Read the model definition and answer for the solid it produces. Units are mm, in the model's axes. Face numbers are marked on the shaded views. A direction names the side the tool comes from. Give positions to 0.01 mm unless a question says otherwise; leave off trailing zeros. Order: outer loops, then holes, each group sorted by start corner. A loop starts at its lowest first (then second) coordinate and runs counter-clockwise, first axis right, second up. Notation, with made-up numbers: (53, 28.25) -> (68, 28.25) arc R29 ccw to (68, 56.25) -> close; hole circle Ø1 at (72.25, 20). An arc over 180 degrees is marked (long way). One line per question, with ' | ' between items. Start each with the question number.
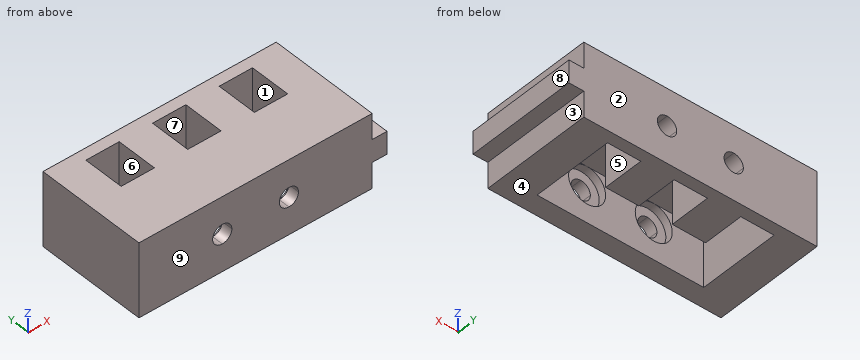
```python
from build123d import *

# Parameters (mm, degrees)
SKETCH_1_W          = 63
SKETCH_1_H          = 30
SKETCH_1_W_2        = 9
SKETCH_1_H_2        = 11
EXTRUDE_2_DEPTH     = 20
SKETCH_2_W          = 9
SKETCH_2_H          = 11
CUT_EXTRUDE_1_DEPTH = 15
SKETCH_3_W          = 9
SKETCH_3_H          = 11
EXTRUDE_3_DEPTH     = 15
CUT_EXTRUDE_2_DEPTH = 100
SKETCH_6_R          = 5
CUT_EXTRUDE_3_DEPTH = 2
SKETCH_7_W          = 3.05
SKETCH_7_H          = 15
EXTRUDE_4_DEPTH     = 4


with BuildPart() as part:
    # 草图1 → 凸台-拉伸2 (new body)
    with BuildSketch(Plane.XY):
        with Locations((18.5, 15)):
            Rectangle(SKETCH_1_W, SKETCH_1_H)
        with Locations((18.5, 21.5)):
            Rectangle(SKETCH_1_W_2, SKETCH_1_H_2, mode=Mode.SUBTRACT)
        with Locations((36.5, 21.5)):
            Rectangle(SKETCH_1_W_2, SKETCH_1_H_2, mode=Mode.SUBTRACT)
        with Locations((0.5, 21.5)):
            Rectangle(SKETCH_1_W_2, SKETCH_1_H_2, mode=Mode.SUBTRACT)
    extrude(amount=EXTRUDE_2_DEPTH)

    # 草图2 → 切除-拉伸1 (cut)
    with BuildSketch(Plane(origin=(0, 0, 0), x_dir=(-1, 0, 0), z_dir=(0, 0, -1))):
        Polygon((-50, 16), (-50, 5), (4, 5), (4, 16), (-5, 16), (-14, 16), (-23, 16), (-32, 16), (-41, 16), align=None)
        with Locations((8.5, 10.5)):
            Rectangle(SKETCH_2_W, SKETCH_2_H)
    extrude(amount=-CUT_EXTRUDE_1_DEPTH, mode=Mode.SUBTRACT)

    # 草图3 → 凸台-拉伸3 (add)
    with BuildSketch(Plane(origin=(0, 0, 0), x_dir=(-1, 0, 0), z_dir=(0, 0, -1))):
        with Locations((-45.5, 10.5)):
            Rectangle(SKETCH_3_W, SKETCH_3_H)
        with Locations((8.5, 10.5)):
            Rectangle(SKETCH_3_W, SKETCH_3_H)
    extrude(amount=-EXTRUDE_3_DEPTH)

    # 草图5 → 切除-拉伸2 (cut)
    with BuildSketch(Plane.XZ):
        with BuildLine():
            ThreePointArc((27.5, 12.6), (25.661522369, 11.838477631), (24.9, 10))
            Line((24.9, 10), (27.5, 10))
            Line((27.5, 10), (27.5, 12.6))
        make_face()
        with BuildLine():
            Line((27.5, 10), (24.9, 10))
            ThreePointArc((24.9, 10), (25.661522369, 8.161522369), (27.5, 7.4))
            Line((27.5, 7.4), (27.5, 10))
        make_face()
        with BuildLine():
            Line((30.1, 10), (27.5, 10))
            Line((27.5, 10), (27.5, 7.4))
            ThreePointArc((27.5, 7.4), (29.338477631, 8.161522369), (30.1, 10))
        make_face()
        with BuildLine():
            Line((27.5, 12.6), (27.5, 10))
            Line((27.5, 10), (30.1, 10))
            ThreePointArc((30.1, 10), (29.338477631, 11.838477631), (27.5, 12.6))
        make_face()
        with BuildLine():
            Line((9.5, 10), (9.5, 7.4))
            ThreePointArc((9.5, 7.4), (11.338477631, 8.161522369), (12.1, 10))
            Line((12.1, 10), (9.5, 10))
        make_face()
        with BuildLine():
            Line((9.5, 12.6), (9.5, 10))
            Line((9.5, 10), (12.1, 10))
            ThreePointArc((12.1, 10), (11.338477631, 11.838477631), (9.5, 12.6))
        make_face()
        with BuildLine():
            ThreePointArc((6.9, 10), (7.661522369, 8.161522369), (9.5, 7.4))
            Line((9.5, 7.4), (9.5, 10))
            Line((9.5, 10), (6.9, 10))
        make_face()
        with BuildLine():
            Line((6.9, 10), (9.5, 10))
            Line((9.5, 10), (9.5, 12.6))
            ThreePointArc((9.5, 12.6), (7.661522369, 11.838477631), (6.9, 10))
        make_face()
    extrude(amount=-CUT_EXTRUDE_2_DEPTH, mode=Mode.SUBTRACT)

    # 草图6 → 切除-拉伸3 (cut)
    with BuildSketch(Plane(origin=(0, 5, 0), x_dir=(1, 0, 0), z_dir=(0, 1, 0))):
        with Locations(Location((9.5, -10, 0), (0, 0, 270))):
            Circle(SKETCH_6_R)
        with Locations(Location((27.5, -10, 0), (0, 0, 270))):
            Circle(SKETCH_6_R)
    extrude(amount=-CUT_EXTRUDE_3_DEPTH, mode=Mode.SUBTRACT)

    # 草图7 → 凸台-拉伸4 (add)
    with BuildSketch(Plane(origin=(50, 0, 0), x_dir=(0, 0, -1), z_dir=(1, 0, 0))):
        with Locations((-8.475, 22.5)):
            Rectangle(SKETCH_7_W, SKETCH_7_H)
        with Locations((-11.525, 22.5)):
            Rectangle(SKETCH_7_W, SKETCH_7_H)
        with Locations((-11.525, 7.5)):
            Rectangle(SKETCH_7_W, SKETCH_7_H)
        with Locations((-8.475, 7.5)):
            Rectangle(SKETCH_7_W, SKETCH_7_H)
    extrude(amount=EXTRUDE_4_DEPTH)


solid = part.part
```
Q1. A cutting plane is placed at C-C, the plane z = 1. Determine the outline of the cut face in (x, y).
Q2. Given P1, Ø2, axis at y = 7, z = 2, coming from the +X side; P2, Ø3, axis at x = 52.5, y = 13.5, coming from the -Z side; P3, Ø1.2, axis at x = 53, y = 15.5, coming from the +Z side, each flat-ended and moving along its own axis, determine where each tip first touches the part or whether it passes through.
Q3. A cutting plane is placed at A-A, the plane y = 25.5. Determine the outline of the cut face in (x, z).
Q4. Which of the six approach directions +Z, -Z, +X, -X, +Y, -Y give full straight-line access (tool end or side, diameter ignored) to the marked faces 1, 2, 3, 4 and 5?
Q5. A cutting plane is placed at B-B, the plane x = 16. Determine the outline of the cut face in (y, z).
Q6. Find the intervals of material crossed by line 1 (X direction, y = 19, z = 7.25); line 2 (X direction, y = 3.5, z = 10); line 3 (Y direction, x = -2.5, z = 5.75), in increasing order.
Q7. A cutting plane is placed at D-D, the plane z = 18.25. Determine the outline of the cut face in (x, y), then the cut area to 3 significant figures.
Q8. Determine the mould class of the marked faces 6, 7, 8 and 9 for opening direction X: pulls with the +X half, pulls with the -X half, needs draft (parallel to the pull), parting line crosses it, or undercut.
Geometry results:
1) outline: (-13, 0) -> (50, 0) -> (50, 30) -> (-13, 30) -> close; hole (-4, 5) -> (41, 5) -> (41, 27) -> (32, 27) -> (32, 16) -> (23, 16) -> (23, 27) -> (14, 27) -> (14, 16) -> (5, 16) -> (5, 27) -> (-4, 27) -> close
2) P1: x = 50 | P2: z = 6.95 | P3: z = 13.05
3) outline: (-13, 0) -> (-4, 0) -> (-4, 20) -> (-13, 20) -> close; (5, 0) -> (14, 0) -> (14, 20) -> (5, 20) -> close; (23, 0) -> (32, 0) -> (32, 20) -> (23, 20) -> close; (41, 0) -> (50, 0) -> (50, 6.95) -> (54, 6.95) -> (54, 13.05) -> (50, 13.05) -> (50, 20) -> (41, 20) -> close; hole circle Ø5.2 at (9.5, 10); hole circle Ø5.2 at (27.5, 10)
4) face 1: -Z | face 2: +Z, -Z, +X, -X, +Y | face 3: -Z, +X, +Y, -Y | face 4: -Z, +X, -X, +Y, -Y | face 5: +Z, -Z
5) outline: (0, 0) -> (5, 0) -> (5, 15) -> (16, 15) -> (16, 20) -> (0, 20) -> close; (27, 0) -> (30, 0) -> (30, 20) -> (27, 20) -> close
6) line 1: -13 to -4, 5 to 14, 23 to 32, 41 to 54 | line 2: -13 to 4.5, 14.5 to 22.5, 32.5 to 54 | line 3: 0 to 5, 27 to 30
7) outline: (-13, 0) -> (50, 0) -> (50, 30) -> (-13, 30) -> close; hole (-4, 16) -> (5, 16) -> (5, 27) -> (-4, 27) -> close; hole (14, 16) -> (23, 16) -> (23, 27) -> (14, 27) -> close; hole (32, 16) -> (41, 16) -> (41, 27) -> (32, 27) -> close | area: 1,590 mm²
8) face 6: undercut | face 7: undercut | face 8: pulls with the +X half | face 9: needs draft
